For this review, use the dimensioned drawing (mm, ordinates from the lowest corner) and the shaded views. A direction names the side the tool comes from. Give positions to 0.01 mm unless a question says otherwise; leave off trailing zeros. Loops run counter-clockwise (first coordinate to the right, second up) from the corner with the lowest first, then second, coordinate; pieces in that order, holes last. Notation, with made-up numbers: (71.5, 10) - (118.5, 10) arc R21 ccw to (118.5, 26) - close; hole circle Ø2 at (-29, 22). An arc over 180 degrees is marked (long way). Put each result on its own line as item: value.
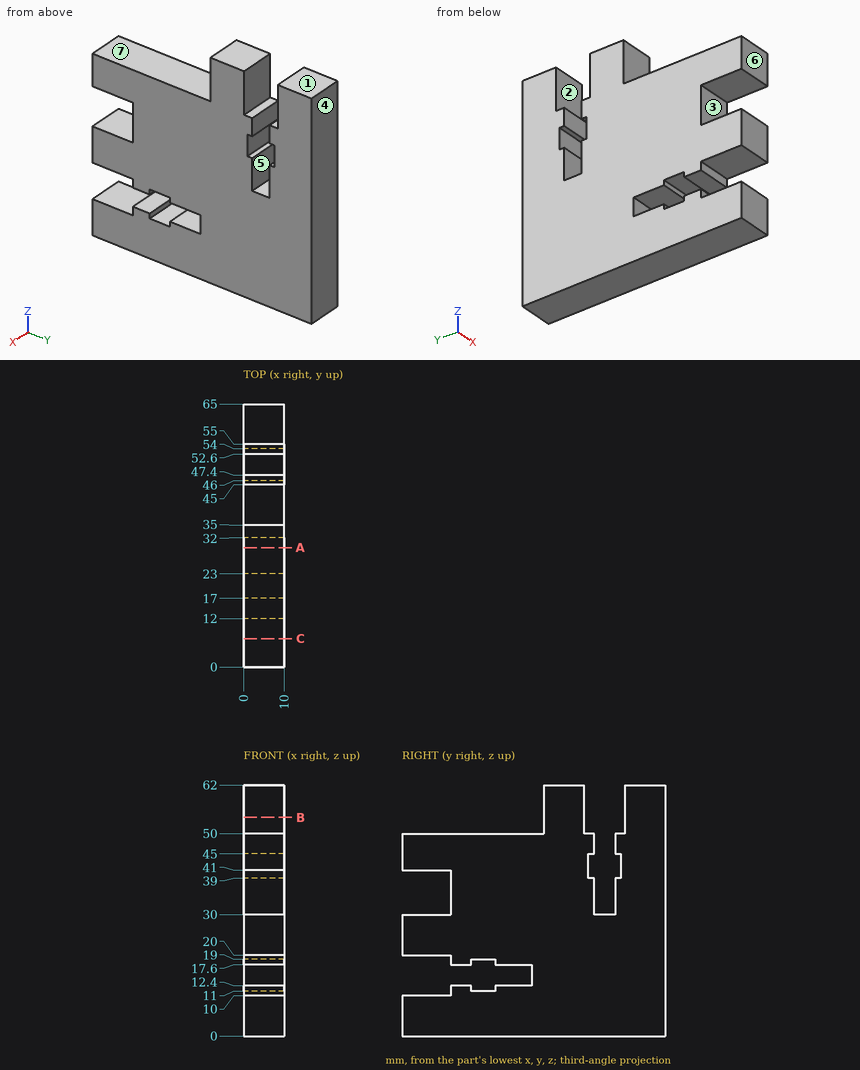
1) Take a section at C-C on y = 7. State the section outline as (x, z) points.
Geometry check:
outline: (0, 0) - (10, 0) - (10, 10) - (0, 10) - close; (0, 20) - (10, 20) - (10, 30) - (0, 30) - close; (0, 41) - (10, 41) - (10, 50) - (0, 50) - close
2) Wall thickness on line 1 (Z direction, x = 8, y = 10); line 2 (Z direction, x = 4, y = 21); line 3 (Y direction, x = 1.25, z = 44): over which ranges is each line inside the solid? List them lowest first.
Geometry check:
line 1: z = 0 to 10, 20 to 30, 41 to 50
line 2: z = 0 to 11, 19 to 50
line 3: y = 0 to 46, 54 to 65
3) For the marked faces 1, 2 and 3, list the 3-axis set-ups (+Z, -Z, +X, -X, +Y, -Y) from which the entire face can be reached by the end or side of a thin tool; tool diameter is ignored.
Geometry check:
face 1: +Z, +X, -X, +Y, -Y
face 2: +Z, +X, -X
face 3: +X, -X, -Y
4) Take a section at B-B on z = 54. State the section outline as (x, y) points, and give its area (3 significant figures).
Geometry check:
outline: (0, 35) - (10, 35) - (10, 45) - (0, 45) - close; (0, 55) - (10, 55) - (10, 65) - (0, 65) - close
area: 200 mm²
5) Take a section at A-A on y = 29.5. State the section outline as (x, z) points.
Geometry check:
outline: (0, 0) - (10, 0) - (10, 12.4) - (0, 12.4) - close; (0, 17.6) - (10, 17.6) - (10, 50) - (0, 50) - close
6) Draft analysis for pull direction Y (two halves, no side actions). For the marked faces 4, 5, 6 and 7, state which applies: pulls with the +Y half, pulls with the -Y half, needs draft (parallel to the pull), parting line crosses it, or undercut.
Geometry check:
face 4: pulls with the +Y half
face 5: undercut
face 6: pulls with the -Y half
face 7: needs draft
7) Insertion check: pin 1 Ø2.5 at (x, z) = (3.5, 47.5) entering from -Y; pin 2 Ø5 at (x, z) = (6.5, 36.5) entering from -Y; pin 3 Ø4 at (x, y) = (3.5, 51) entering from +Z. Each pin has a flat end and moves straight along its axis. Give the tip position at first contact, or say it passes through.
Geometry check:
pin 1: stops at y = 0
pin 2: stops at y = 12
pin 3: stops at z = 50
